Autodesk Inventor part; units mm, degrees
ref_plane "YZ Plane" through (0, 0, 0) normal (1, 0, 0) x (0, 1, 0)
ref_plane "XZ Plane" through (0, 0, 0) normal (0, 1, 0) x (-1, 0, 0)
ref_plane "XY Plane" through (0, 0, 0) normal (0, 0, 1) x (1, 0, 0)
sketch "スケッチ1" plane through (0, 0, 0) normal (0, 0, 1) x (1, 0, 0)
  line L0 (-16, 21.5) -> (-10.583, 21.5) construction
  line L1 (16, 21.5) -> (16, 9.5) construction
  line L2 (16, -21.5) -> (-16, -21.5)
  line L3 (-16, -21.5) -> (-16, 9.5)
  line L4 (-16, 21.5) -> (16, -21.5) construction
  line L5 (16, 21.5) -> (-16, -21.5) construction
  line L6 (-14.4, -21.5) -> (-14.4, -30)
  line L7 (-14.4, -30) -> (14.4, -30)
  line L8 (0, 21.5) -> (0, -21.5) construction
  line L9 (14.4, -21.5) -> (14.4, -30)
  line L10 (-13.5, 21.5) -> (-13.5, -21.5) construction
  circle A0 centre (0, 9.5) radius 6
  circle A1 centre (0, 9.5) radius 4
  arc A2 (-10.583, 21.5) -> (-16, 9.5) centre (0, 9.5) ccw
  arc A3 (16, 9.5) -> (10.583, 21.5) centre (0, 9.5) ccw
  line L11 (-10.583, 21.5) -> (10.583, 21.5)
  line L12 (-16, 9.5) -> (-16, 21.5) construction
  line L13 (10.583, 21.5) -> (16, 21.5) construction
  line L14 (16, 9.5) -> (16, -21.5)
  circle A4 centre (0, 9.5) radius 3
  circle A5 centre (0, 9.5) radius 4.8
  point P0 (0, 0)
  point P1 (-13.5, 8.5)
  point P2 (-13.5, -18.5)
  point P3 (13.5, 8.5)
  point P4 (13.5, -18.5)
  dimension "d0" = 32
  dimension "d1" = 43
  dimension "d4" = 28.8
  dimension "d5" = 8.5
  dimension "d8" = 27
  dimension "d9" = 8.5
  dimension "d12" = 18.5
  dimension "d13" = 12
  dimension "d14" = 8
  dimension "d15" = 9.5
  dimension "d17" = 16
  dimension "d32" = 13.5
  dimension "d47" = 6
  dimension "d67" = 9.6
extrude "押し出し1" add sketch "スケッチ1" against normal blind 12.2 contours L2 L3 A2 L11 A3 L14 | A0 | A1 | A4 | A5
extrude "押し出し2" add sketch "スケッチ1" against normal blind 12 contours L9 L7 L6 L2
extrude "押し出し3" add sketch "スケッチ1" against normal blind 14 contours A0 | A1 | A4 | A5
extrude "押し出し4" add sketch "スケッチ1" against normal blind 17.7 contours A1 | A4
chamfer "面取り1" distance 1.2 angle 45 1 edges at (-6, 9.5, -14)
sketch "スケッチ2" plane through (0, 9.5, -17.7) normal (0, 0, -1) x (-1, 0, 0)
  circle A0 centre (0, 0) radius 4
  point P0 (0, -9.5)
hole "穴1" at (0, 9.5, -17.7) direction (0, 0, 1) diameter 2.459 depth 6
extrude "押し出し5" add sketch "スケッチ1" along normal blind 20.3 contours L2 L3 A2 L11 A3 L14 | A0 | A1 | A4 | A5
hole "穴2" at (-13.5, 8.5, 0) at (-13.5, -18.5, 0) at (13.5, 8.5, 0) at (13.5, -18.5, 0) direction (0, 0, 1) diameter 2.7 end through all both
extrude "押し出し6" cut sketch "スケッチ1" against normal blind 0.4 contours L9 L7 L6 L2
fillet "フィレット1" radius 2 2 edges at (16, -21.5, 4.05) (-16, -21.5, 4.05)
extrude "押し出し7" add sketch "スケッチ1" along normal blind 20.8 contours A0 | A1 | A4 | A5
extrude "押し出し8" add sketch "スケッチ1" along normal blind 23.75 contours A4
sketch "スケッチ3" plane through (0, 9.5, 23.75) normal (0, 0, 1) x (1, 0, 0)
  circle A0 centre (0, 0) radius 1.2295
  point P0 (0, -9.5)
hole "穴3" at (0, 9.5, 23.75) direction (0, 0, -1) diameter 2.459 end through all
sketch "スケッチ4" plane through (0, 9.5, 20.8) normal (0, 0, 1) x (1, 0, 0)
  circle A0 centre (0, 0) radius 4
  circle A1 centre (0, 0) radius 3
  point P0 (0, -9.5)
extrude "押し出し9" cut sketch "スケッチ4" against normal blind 2.3
chamfer "面取り2" distance 0.5 angle 45 1 edges at (-3, 9.5, 23.75)
extrude "押し出し10" add sketch "スケッチ1" against normal blind 14.2 contours A5
properties part number "B3M10xx"
Check sheet for the modelled part. Datum: model origin and axes. Units: mm. A direction names the side the tool comes from. Coordinates: 2 decimals unless noted, no trailing zeros. Write each loop counter-clockwise with the first axis right and the second up, starting at its lowest first coordinate (ties: lowest second). Pieces come first, ordered by that corner, then holes. Notation, with made-up numbers: M 28,-9 L 69,-9 A18 cw 69,4 Z; hole C -16,29.5 d6. An arc over 180 degrees is marked long. Use one line per item in the form item = value.
Item 1: Release check for a two-part mould opening along X. For faces 5 (the face through (14.62, 16, 4.28)), 6 (the face through (-15.43, -20.9, 4.28)), 7 (the face through (-0.391, 6.526, 20.842)), 8 (the face through (4, 8, 20.8)) record: pulls with the +X half, pulls with the -X half, needs draft (parallel to the pull), parting line crosses it, or undercut.
Answer below:
face_5 = pulls with the +X half
face_6 = pulls with the -X half
face_7 = undercut
face_8 = needs draft
Item 2: Material ranges on L1, parallel to Y at x = 0, z = 19.1; L2, parallel to X at y = -18.5, z = 11.5; L3, parallel to Y at x = 0, z = -6, recorded low to high. Write a range as from..to.
Answer below:
L1 = -21.5..5.5, 6.5..8.27, 10.73..12.5, 13.5..21.5
L2 = -16..-14.85, -12.15..12.15, 14.85..16
L3 = -30..8.27, 10.73..21.5
Item 3: Set-up check for faces 1 (the face through (-1.301, 3.643, -12.496)), 2 (the face through (3.815, 10.701, 19.666)), 3 (the face through (0, -26, -0.4)), 4 (the face through (-14.4, -26, -6)): record each of +Z, -Z, +X, -X, +Y, -Y from which the full face is reachable in a straight line by a thin tool's end or side.
Answer below:
face_1 = -Z
face_2 = +Z
face_3 = +Z, +X, -X, -Y
face_4 = +Z, -Z, -X, -Y
Item 4: Sectioned sample at B-B, the plane y = -18.5. Record the cut outline in (x, z).
Answer below:
outline = M -16,-12.2 L -14.85,-12.2 L -14.85,20.3 L -16,20.3 Z; M -12.15,-12.2 L 12.15,-12.2 L 12.15,20.3 L -12.15,20.3 Z; M 14.85,-12.2 L 16,-12.2 L 16,20.3 L 14.85,20.3 Z
Item 5: Sectioned sample at C-C, the plane x = -11.5. Record the cut outline in (y, z).
Answer below:
outline = M -30,-12 L -21.5,-12 L -21.5,-12.2 L 20.62,-12.2 L 20.62,20.3 L -21.5,20.3 L -21.5,-0.4 L -30,-0.4 Z
Item 6: Sectioned sample at A-A, the plane z = 8. Record the cut outline in (x, y).
Answer below:
outline = M -16,-19.5 A2 ccw -14,-21.5 L 14,-21.5 A2 ccw 16,-19.5 L 16,9.5 A16 ccw 10.58,21.5 L -10.58,21.5 A16 ccw -16,9.5 Z; hole C -13.5,-18.5 d2.7; hole C -13.5,8.5 d2.7; hole C 0,9.5 d2.46; hole C 13.5,-18.5 d2.7; hole C 13.5,8.5 d2.7
Item 7: Gauge pin test, flat ends, axial feed: pin 1 Ø9.5 at (x, y) = (6, -0.5) entering from +Z; pin 2 Ø1 at (x, z) = (12.5, 19) entering from -Y; pin 3 Ø4.5 at (x, y) = (-6, -26) entering from +Z. Record the tip position at first contact, or that the pin passes through.
Answer below:
pin_1 = 20.3
pin_2 = -21.5
pin_3 = -0.4
